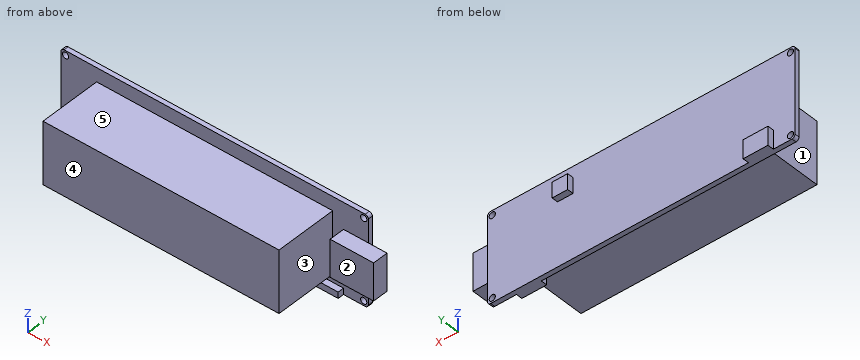
Autodesk Inventor part; units mm, degrees
ref_plane "YZ Plane" through (0, 0, 0) normal (1, 0, 0) x (0, 1, 0)
ref_plane "XZ Plane" through (0, 0, 0) normal (0, 1, 0) x (-1, 0, 0)
ref_plane "XY Plane" through (0, 0, 0) normal (0, 0, 1) x (1, 0, 0)
sketch "Sketch1" plane through (0, 0, 0) normal (0, 1, 0) x (-1, 0, 0)
  line L0 (49.5, 14.5) -> (-49.5, 14.5)
  line L1 (-49.5, 14.5) -> (-49.5, -14.5)
  line L2 (-49.5, -14.5) -> (49.5, -14.5)
  line L3 (49.5, -14.5) -> (49.5, 14.5)
  line L4 (49.5, 14.5) -> (-49.5, -14.5) construction
  line L5 (-49.5, 14.5) -> (49.5, -14.5) construction
  point P0 (0, 0)
  dimension "d0" = 99
  dimension "d1" = 29
extrude "Extrusion1" add sketch "Sketch1" along normal blind 1.5
fillet "Fillet1" radius 1 4 edges at (49.5, 0.75, 14.5) (49.5, 0.75, -14.5) (-49.5, 0.75, -14.5) (-49.5, 0.75, 14.5)
sketch "Sketch2" plane through (0, 1.5, 0) normal (0, 1, 0) x (1, 0, 0)
  line L0 (26.9904, -10.9774) -> (21.9904, -10.9774)
  line L1 (21.9904, -10.9774) -> (21.9904, -5.9774)
  line L2 (21.9904, -5.9774) -> (26.9904, -5.9774)
  line L3 (26.9904, -5.9774) -> (26.9904, -10.9774)
  line L4 (26.9904, -10.9774) -> (21.9904, -5.9774) construction
  line L5 (21.9904, -10.9774) -> (26.9904, -5.9774) construction
  point P0 (0, 0)
  point P1 (24.4904, -8.4774)
  dimension "d5" = 5
  dimension "d6" = 5
extrude "Extrusion2" add sketch "Sketch2" along normal blind 2
sketch "Sketch3" plane through (0, 1.5, 0) normal (0, 1, 0) x (1, 0, 0)
  line L0 (26.9904, -5.9774) -> (26.9904, -10.9774) construction
  line L1 (26.9904, -10.9774) -> (21.9904, -10.9774) construction
  line L2 (21.9904, -10.9774) -> (21.9904, -5.9774) construction
  line L3 (21.9904, -5.9774) -> (26.9904, -5.9774) construction
  arc A0 (-49.5, -13.5) -> (-48.5, -14.5) centre (-48.5, -13.5) ccw construction
  line L4 (-48.5, -14.5) -> (48.5, -14.5) construction
  arc A1 (48.5, -14.5) -> (49.5, -13.5) centre (48.5, -13.5) ccw construction
  line L5 (49.5, -13.5) -> (49.5, 13.5) construction
  arc A2 (49.5, 13.5) -> (48.5, 14.5) centre (48.5, 13.5) ccw construction
  line L6 (48.5, 14.5) -> (-48.5, 14.5) construction
  arc A3 (-48.5, 14.5) -> (-49.5, 13.5) centre (-48.5, 13.5) ccw construction
  line L7 (-49.5, 13.5) -> (-49.5, -13.5) construction
  line L8 (48, -13) -> (-48, -13) construction
  line L9 (-48, -13) -> (-48, 13) construction
  line L10 (-48, 13) -> (48, 13) construction
  line L11 (48, 13) -> (48, -13) construction
  point P0 (0, 0)
  dimension "d9" = 1.5
hole "Hole1" at (48, 1.5, 13) at (-48, 1.5, 13) at (-48, 1.5, -13) at (48, 1.5, -13) direction (0, -1, 0) diameter 2 depth 10 tip angle 118
sketch "Sketch4" plane through (0, 1.5, 0) normal (0, 1, 0) x (1, 0, 0)
  line L0 (-49.5, 13.5) -> (-49.5, -13.5) construction
  line L1 (-49.5, 10.3219) -> (-42.5, 10.3219) construction
  line L2 (-34.5, 8.5) -> (-42.5, 8.5)
  line L3 (-42.5, 8.5) -> (-42.5, 14.5)
  line L4 (-42.5, 14.5) -> (-34.5, 14.5)
  line L5 (-34.5, 14.5) -> (-34.5, 8.5)
  line L6 (-34.5, 8.5) -> (-42.5, 14.5) construction
  line L7 (-42.5, 8.5) -> (-34.5, 14.5) construction
  line L8 (48.5, 14.5) -> (-48.5, 14.5) construction
  point P0 (0, 0)
  point P1 (-38.5, 11.5)
  dimension "d17" = 7
  dimension "d18" = 8
  dimension "d19" = 6
extrude "Extrusion3" add sketch "Sketch4" along normal blind 2
sketch "Sketch5" plane through (0, 1.5, 0) normal (0, 1, 0) x (1, 0, 0)
  line L0 (49.5, -13.5) -> (49.5, 13.5) construction
  line L1 (49.5, 9.2214) -> (41.5, 9.2214) construction
  line L2 (48.5, 14.5) -> (-34.5, 14.5) construction
  line L3 (41.5, 12.5) -> (33.5, 12.5)
  line L4 (33.5, 12.5) -> (33.5, 14.5)
  line L5 (33.5, 14.5) -> (41.5, 14.5)
  line L6 (41.5, 14.5) -> (41.5, 12.5)
  line L7 (41.5, 12.5) -> (33.5, 14.5) construction
  line L8 (33.5, 12.5) -> (41.5, 14.5) construction
  point P0 (0, 0)
  point P1 (37.5, 13.5)
  dimension "d22" = 8
  dimension "d23" = 8
  dimension "d24" = 2
sketch "Sketch6" plane through (0, 0, 0) normal (0, -1, 0) x (1, 0, 0)
  line L0 (41.5, -12.5) -> (33.5, -12.5)
  line L1 (41.5, -14.5) -> (41.5, -12.5)
  line L2 (33.5, -12.5) -> (33.5, -14.5)
  line L3 (41.5, -14.5) -> (33.5, -14.5)
  point P0 (0, 0)
extrude "Extrusion4" add sketch "Sketch6" along normal blind 2
sketch "Sketch7" plane through (0, 0, 0) normal (0, -1, 0) x (1, 0, 0)
  line L0 (33.5, -14.5) -> (33.5, -12.5) construction
  line L1 (33.5, -12.5) -> (41.5, -12.5) construction
  line L2 (41.5, -12.5) -> (41.5, -14.5) construction
  line L3 (48.5, -14.5) -> (41.5, -14.5) construction
  arc A0 (48.5, -14.5) -> (49.5, -13.5) centre (48.5, -13.5) ccw construction
  line L4 (49.5, 13.5) -> (49.5, -13.5) construction
  arc A1 (49.5, 13.5) -> (48.5, 14.5) centre (48.5, 13.5) ccw construction
  line L5 (-48.5, 14.5) -> (48.5, 14.5) construction
  arc A2 (-48.5, 14.5) -> (-49.5, 13.5) centre (-48.5, 13.5) ccw construction
  line L6 (-49.5, -13.5) -> (-49.5, 13.5) construction
  arc A3 (-49.5, -13.5) -> (-48.5, -14.5) centre (-48.5, -13.5) ccw construction
  line L7 (33.5, -14.5) -> (-48.5, -14.5) construction
  circle A4 centre (48, -13) radius 1 construction
  circle A5 centre (-48, 13) radius 1 construction
  circle A6 centre (48, 13) radius 1 construction
  circle A7 centre (-48, -13) radius 1 construction
  line L8 (55.5, -6) -> (41.5, -6)
  line L9 (41.5, -6) -> (41.5, 6)
  line L10 (41.5, 6) -> (55.5, 6)
  line L11 (55.5, 6) -> (55.5, -6)
  line L12 (55.5, -6) -> (41.5, 6) construction
  line L13 (41.5, -6) -> (55.5, 6) construction
  line L14 (49.5, 0) -> (55.5, 0) construction
  point P0 (0, 0)
  point P1 (48.5, 0)
  dimension "d27" = 14
  dimension "d28" = 12
  dimension "d29" = 6
extrude "Extrusion5" add sketch "Sketch7" along normal blind 5
sketch "Sketch8" plane through (0, 0, 0) normal (0, -1, 0) x (1, 0, 0)
  line L0 (41.5, 6) -> (49.5, 6) construction
  line L1 (49.5, 13.5) -> (49.5, 6) construction
  arc A0 (49.5, 13.5) -> (48.5, 14.5) centre (48.5, 13.5) ccw construction
  line L2 (-48.5, 14.5) -> (48.5, 14.5) construction
  arc A1 (-48.5, 14.5) -> (-49.5, 13.5) centre (-48.5, 13.5) ccw construction
  line L3 (-49.5, -13.5) -> (-49.5, 13.5) construction
  arc A2 (-49.5, -13.5) -> (-48.5, -14.5) centre (-48.5, -13.5) ccw construction
  line L4 (33.5, -14.5) -> (-48.5, -14.5) construction
  line L5 (33.5, -14.5) -> (33.5, -12.5) construction
  line L6 (33.5, -12.5) -> (41.5, -12.5) construction
  line L7 (41.5, -12.5) -> (41.5, -14.5) construction
  line L8 (48.5, -14.5) -> (41.5, -14.5) construction
  arc A3 (48.5, -14.5) -> (49.5, -13.5) centre (48.5, -13.5) ccw construction
  line L9 (49.5, -6) -> (49.5, -13.5) construction
  line L10 (49.5, -6) -> (41.5, -6) construction
  line L11 (41.5, -6) -> (41.5, 6) construction
  circle A4 centre (48, -13) radius 1 construction
  circle A5 centre (-48, 13) radius 1 construction
  circle A6 centre (48, 13) radius 1 construction
  circle A7 centre (-48, -13) radius 1 construction
  line L12 (38, -10) -> (-38, -10)
  line L13 (-38, -10) -> (-38, 10)
  line L14 (-38, 10) -> (38, 10)
  line L15 (38, 10) -> (38, -10)
  line L16 (38, -10) -> (-38, 10) construction
  line L17 (-38, -10) -> (38, 10) construction
  point P0 (0, 0)
  point P1 (0, 0)
  point P2 (0, 0)
  dimension "d32" = 76
  dimension "d33" = 20
extrude "Extrusion6" add sketch "Sketch8" along normal blind 20
properties part number "battery_footprint"
Geometry check sheet. Reference: the model listing, model coordinates, mm. Face numbers are marked on the shaded views. A direction names the side the tool comes from. Coordinates: 2 decimals unless noted, no trailing zeros. Order: outer loops, then holes, each group sorted by start corner. A loop starts at its lowest first (then second) coordinate and runs counter-clockwise, first axis right, second up. Notation, with made-up numbers: M -30,-15.75 L -1,-15.75 A21 cw -1,-3.75 Z; hole C 64.25,9 d7. An arc over 180 degrees is marked long. One line per question, with ' | ' between items. Start each with the question number.
Item 1: Material ranges on L1, parallel to Z at x = -48, y = 1; L2, parallel to X at y = 0.7, z = -13; L3, parallel to Y at x = -32, z = 4.25, recorded low to high. Write a range as [from, to].
Item 2: Draft check along X on the marked faces 1, 2 and 3. Enter one of: pulls with the +X half, pulls with the -X half, needs draft (parallel to the pull), parting line crosses it, or undercut.
Item 3: Cross-section at A-A on y = -3.25. Enter the section's corners in (x, z), then the cut area to 3 significant figures.
Item 4: Set-up check for the marked faces 4 and 5: record each of +Z, -Z, +X, -X, +Y, -Y from which the full face is reachable in a straight line by a thin tool's end or side.
Item 5: Gauge pin test, flat ends, axial feed: pin 1 (1 mm diameter, centred on x = -29, y = -6.5, fed in from -Z); pin 2 (4 mm diameter, centred on y = -10.5, z = 3.5, fed in from -X); pin 3 (1.8 mm diameter, centred on x = 54, z = 2.5, fed in from +Y); pin 4 (1.2 mm diameter, centred on x = 48, z = -13, fed in from -Y). Record the tip position at first contact, or that the pin passes through.
Item 6: Cross-section at B-B on x = -5. Enter the section's corners in (y, z), then the cut area to 4 significant figures.
Item 7: Cross-section at C-C on z = -4.75. Enter the section's corners in (x, y), then the cut area to 3 significant figures.
Item 8: Cross-section at D-D on x = -40. Enter the section's corners in (y, z), then the cut area to 3 significant figures.
Findings:
1) L1: z = [-14.5, -14], [-12, 12], [14, 14.5] | L2: x = [-49.5, -49], [-47, 47], [49, 49.5] | L3: y = [-20, 1.5]
2) face 1: pulls with the -X half | face 2: needs draft | face 3: undercut
3) outline: M -38,-10 L 38,-10 L 38,10 L -38,10 Z; M 41.5,-6 L 55.5,-6 L 55.5,6 L 41.5,6 Z | area: 1,690 mm²
4) face 4: +Z, -Z, +X, -X, -Y | face 5: +Z, +X, -X, -Y
5) pin 1: stops at z = -10 | pin 2: stops at x = -38 | pin 3: stops at y = 0 | pin 4: passes through
6) outline: M -20,-10 L 0,-10 L 0,-14.5 L 1.5,-14.5 L 1.5,14.5 L 0,14.5 L 0,10 L -20,10 Z | area: 443.5 mm²
7) outline: M -49.5,0 L -38,0 L -38,-20 L 38,-20 L 38,0 L 41.5,0 L 41.5,-5 L 55.5,-5 L 55.5,0 L 49.5,0 L 49.5,1.5 L -49.5,1.5 Z | area: 1,740 mm²
8) outline: M 0,-14.5 L 3.5,-14.5 L 3.5,-8.5 L 1.5,-8.5 L 1.5,14.5 L 0,14.5 Z | area: 55.5 mm²
